Geometry check sheet. Reference: the model listing, model coordinates, mm. Face numbers are marked on the shaded views. Round coordinates to 2 decimals unless told otherwise and drop trailing zeros. Order: outer loops, then holes, each group sorted by start corner. A loop starts at its lowest first (then second) coordinate and runs counter-clockwise, first axis right, second up.
```python
from build123d import *
from OCP.BRepFilletAPI import BRepFilletAPI_MakeChamfer

# Parameters (mm, degrees)
SKETCH2_W                = 6.219952
SKETCH2_H                = 2.794
BASE_EXTRUDE_DEPTH       = 7.10946
CHAMFER1_SIZE            = 1.397
CHAMFER1_SIZE2           = 0.246328792
SKETCH3_W                = 3.556
SKETCH3_H                = 1.27
CUT_EXTRUDE1_DEPTH       = 0.508
SKETCH4_W                = 3.556
SKETCH4_H                = 1.27
CUT_EXTRUDE2_DEPTH       = 0.508
SKETCH5_OUTSIDE_W        = 11.079
SKETCH5_OUTSIDE_H        = 10.19
SKETCH5_OUTSIDE_W_2      = 3.302
SKETCH5_OUTSIDE_H_2      = 3.600196
CUT_EXTRUDE3_DEPTH       = 0.254
CHAMFER2_SIZE            = 1.397
CHAMFER2_SIZE_2          = 0.246328792
BOSS_EXTRUDE_THIN1_DEPTH = 1.589913
SKETCH7_W                = 1.524
SKETCH7_H                = 0.381
CUT_EXTRUDE4_DEPTH       = 0.508
SKETCH8_W                = 1.35763
SKETCH8_H                = 5.727294416
BOSS_EXTRUDE2_DEPTH      = 0.00254


with BuildPart() as part:
    # Sketch2 → Base-Extrude (new body)
    with BuildSketch(Plane(origin=(0, 0, 0), x_dir=(0, 0, -1), z_dir=(1, 0, 0))):
        with Locations((0, 1.397)):
            Rectangle(SKETCH2_W, SKETCH2_H)
    extrude(amount=BASE_EXTRUDE_DEPTH)

    # Chamfer1: one chamfer whose edges measure the first distance from different faces: ONE call of the kernel's chamfer builder (chamfer() names one face for all edges)
    chamfer1_edges_1 = [part.edges().sort_by_distance(p)[0] for p in [
        (7.10946, 0, 0),
    ]]
    chamfer1_side_1 = [part.faces().sort_by_distance(p)[0] for p in [
        (7.10946, 1.397, 0),
    ]]
    chamfer1_edges_2 = [part.edges().sort_by_distance(p)[0] for p in [
        (0, 0, 0),
    ]]
    chamfer1_side_2 = [part.faces().sort_by_distance(p)[0] for p in [
        (0, 1.397, 0),
    ]]
    chamfer1_edges_3 = [part.edges().sort_by_distance(p)[0] for p in [
        (3.55473, 0, -3.109976),
    ]]
    chamfer1_side_3 = [part.faces().sort_by_distance(p)[0] for p in [
        (3.55473, 1.397, -3.109976),
    ]]
    chamfer1_edges_4 = [part.edges().sort_by_distance(p)[0] for p in [
        (3.55473, 0, 3.109976),
    ]]
    chamfer1_side_4 = [part.faces().sort_by_distance(p)[0] for p in [
        (3.55473, 1.397, 3.109976),
    ]]
    chamfer1 = BRepFilletAPI_MakeChamfer(part.part.solid().wrapped)
    for e in chamfer1_edges_1:
        chamfer1.Add(CHAMFER1_SIZE, CHAMFER1_SIZE2, e.wrapped, chamfer1_side_1[0].wrapped)  # the first distance lies on this face
    for e in chamfer1_edges_2:
        chamfer1.Add(CHAMFER1_SIZE, CHAMFER1_SIZE2, e.wrapped, chamfer1_side_2[0].wrapped)  # the first distance lies on this face
    for e in chamfer1_edges_3:
        chamfer1.Add(CHAMFER1_SIZE, CHAMFER1_SIZE2, e.wrapped, chamfer1_side_3[0].wrapped)  # the first distance lies on this face
    for e in chamfer1_edges_4:
        chamfer1.Add(CHAMFER1_SIZE, CHAMFER1_SIZE2, e.wrapped, chamfer1_side_4[0].wrapped)  # the first distance lies on this face
    add(Compound.cast(chamfer1.Shape()), mode=Mode.REPLACE)

    # Sketch3 → Cut-Extrude1 (cut)
    with BuildSketch(Plane.ZY):
        with Locations((0, 0.635)):
            Rectangle(SKETCH3_W, SKETCH3_H)
    extrude(amount=-CUT_EXTRUDE1_DEPTH, mode=Mode.SUBTRACT)

    # Sketch4 → Cut-Extrude2 (cut)
    with BuildSketch(Plane(origin=(7.10946, 0, 0), x_dir=(0, 0, -1), z_dir=(1, 0, 0))):
        with Locations((0, 0.635)):
            Rectangle(SKETCH4_W, SKETCH4_H)
    extrude(amount=-CUT_EXTRUDE2_DEPTH, mode=Mode.SUBTRACT)

    # Sketch5 outside → Cut-Extrude3 (cut)
    with BuildSketch(Plane.XZ):
        with Locations((3.5545, 0)):
            Rectangle(SKETCH5_OUTSIDE_W, SKETCH5_OUTSIDE_H)
        with Locations((3.556, 0)):
            Rectangle(SKETCH5_OUTSIDE_W_2, SKETCH5_OUTSIDE_H_2, mode=Mode.SUBTRACT)
    extrude(amount=-CUT_EXTRUDE3_DEPTH, mode=Mode.SUBTRACT)

    # Chamfer2
    chamfer2_edges_1 = [part.edges().sort_by_distance(p)[0] for p in [
        (0, 2.794, 0),
    ]]
    chamfer2_side_1 = [part.faces().sort_by_distance(p)[0] for p in [
        (0, 2.789073424, 0),
    ]]
    chamfer2_edges_2 = [part.edges().sort_by_distance(p)[0] for p in [
        (7.10946, 2.794, 0),
    ]]
    chamfer2_side_2 = [part.faces().sort_by_distance(p)[0] for p in [
        (7.104533424, 2.794, 0),
    ]]
    chamfer2_edges_3 = [part.edges().sort_by_distance(p)[0] for p in [
        (3.55473, 2.794, 3.109976),
    ]]
    chamfer2_side_3 = [part.faces().sort_by_distance(p)[0] for p in [
        (3.55473, 2.789073424, 3.109976),
    ]]
    chamfer2_edges_4 = [part.edges().sort_by_distance(p)[0] for p in [
        (3.55473, 2.794, -3.109976),
    ]]
    chamfer2_side_4 = [part.faces().sort_by_distance(p)[0] for p in [
        (3.55473, 2.794, -3.105049424),
    ]]
    chamfer2 = BRepFilletAPI_MakeChamfer(part.part.solid().wrapped)
    for e in chamfer2_edges_1:
        chamfer2.Add(CHAMFER2_SIZE - 0.0001, CHAMFER2_SIZE_2 - 0.0001, e.wrapped, chamfer2_side_1[0].wrapped)
    for e in chamfer2_edges_2:
        chamfer2.Add(CHAMFER2_SIZE_2 - 0.0001, CHAMFER2_SIZE - 0.0001, e.wrapped, chamfer2_side_2[0].wrapped)
    for e in chamfer2_edges_3:
        chamfer2.Add(CHAMFER2_SIZE - 0.0001, CHAMFER2_SIZE_2 - 0.0001, e.wrapped, chamfer2_side_3[0].wrapped)
    for e in chamfer2_edges_4:
        chamfer2.Add(CHAMFER2_SIZE_2 - 0.0001, CHAMFER2_SIZE - 0.0001, e.wrapped, chamfer2_side_4[0].wrapped)
    add(Compound.cast(chamfer2.Shape()), mode=Mode.REPLACE)  # a hair under: the kernel refuses the full size

    # Sketch6 → Boss-Extrude-Thin1 (add, symmetric)
    with BuildSketch(Plane.XY):
        Polygon((0.295515086, 1.267447171), (-0.002552829, 1.267447171), (-0.254, 1.016), (-0.254, 0.254), (0, 0), (1.2954, 0), (1.2954, 0.254), (0.105210245, 0.254), (0, 0.359210245), (0, 0.910789755), (0.102657416, 1.013447171), (0.295515086, 1.013447171), align=None)
    boss_extrude_thin1 = extrude(amount=BOSS_EXTRUDE_THIN1_DEPTH, both=True)

    # Sketch7 → Cut-Extrude4 (cut)
    with BuildSketch(Plane.ZY.offset(0.254)):
        with Locations((0, 1.0795)):
            Rectangle(SKETCH7_W, SKETCH7_H)
    cut_extrude4 = extrude(amount=-CUT_EXTRUDE4_DEPTH, mode=Mode.SUBTRACT)

    # Mirror1: Boss-Extrude-Thin1, Cut-Extrude4 across plane
    add(boss_extrude_thin1.mirror(Plane(origin=(3.554984, 0, 0), x_dir=(0, 0, 1), z_dir=(1, 0, 0))))
    add(cut_extrude4.mirror(Plane(origin=(3.554984, 0, 0), x_dir=(0, 0, 1), z_dir=(1, 0, 0))), mode=Mode.SUBTRACT)

    # Sketch8 → Boss-Extrude2 (add)
    with BuildSketch(Plane(origin=(0, 2.794, 0), x_dir=(-1, 0, 0), z_dir=(0, 1, 0))):
        with Locations((-6.078855, 0)):
            Rectangle(SKETCH8_W, SKETCH8_H)
    extrude(amount=BOSS_EXTRUDE2_DEPTH)


solid = part.part
```
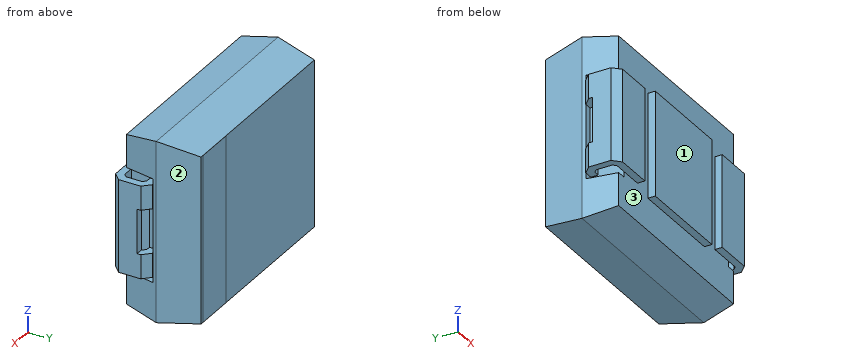
(1) Sectioned sample at D-D, the plane z = 0. Give the number of separate pieces and of enclosed holes in the cut face, and give its area (3 significant figures).
Returned:
separate pieces: 3
enclosed holes: 0
area: 18.6 mm2
(2) Material ranges on line 1 (X direction, y = 0.55, z = 0.5); line 2 (X direction, y = 0.2, z = -1.5) (3 decimals); line 3 (Y direction, x = 6.5, z = 2.5), recorded low to high.
Returned:
line 1: x = -0.25 to 0, 0.51 to 6.6, 7.11 to 7.36
line 2: x = -0.2 to 1.295, 1.905 to 5.207, 5.815 to 7.31
line 3: y = 0.25 to 2.8
(3) Sectioned sample at B-B, the plane y = 1.1. Record the cut outline in (x, z), and give its area (3 significant figures).
Returned:
outline: (-0.17, -1.59) - (0.3, -1.59) - (0.3, 1.59) - (-0.17, 1.59) - (-0.17, 0.76) - (0.25, 0.76) - (0.25, -0.76) - (-0.17, -0.76) - close; (0.05, -3.06) - (7.06, -3.06) - (7.06, -1.78) - (6.6, -1.78) - (6.6, 1.78) - (7.06, 1.78) - (7.06, 3.06) - (0.05, 3.06) - (0.05, 1.78) - (0.51, 1.78) - (0.51, -1.78) - (0.05, -1.78) - close; (6.81, -1.59) - (7.28, -1.59) - (7.28, -0.76) - (6.86, -0.76) - (6.86, 0.76) - (7.28, 0.76) - (7.28, 1.59) - (6.81, 1.59) - close
area: 41.3 mm2
(4) Draft check along X on the marked faces 1, 2 and 3. Enter one of: released by +X, released by -X, zero draft, split by the parting line, or undercut.
Returned:
face 1: zero draft
face 2: released by +X
face 3: undercut
(5) Depth check by flat-ended pin: P1, Ø1.5, axis at y = 2, z = -2, coming from the -X side; P2, Ø0.5, axis at x = 0.5, y = 0.5, coming from the -Z side. Enter the tip coordinate at first touch or a pass-through.
Returned:
P1: stops at x = 0
P2: stops at z = -3
